```python
from build123d import *

# Parameters (mm, degrees)
MOUNTING_POINTS_DEPTH      = 116.951759253
MOUNTING_POINTS_DEPTH_BACK = 116.951759253
SKETCH3_R                  = 4.25
SKETCH3_R_2                = 12
SLOT_CLEARANCE_DEPTH       = 116.951759253
SLOT_CLEARANCE_DEPTH_BACK  = 116.951759253


with BuildPart() as part:
    # Sweep1: sweep along a path in Sketch1
    with BuildLine(Plane(origin=(0, 0, 0), x_dir=(1, 0, 0), z_dir=(0, 1, 0))) as sweep1_path:
        ThreePointArc((-100, -5), (0, 0), (100, -5))
    # Sketch2 → Sweep1 (sweep)
    with BuildSketch(Plane(origin=(0, 0, 0), x_dir=(0, 0, -1), z_dir=(1, 0, 0))):
        with BuildLine():
            Line((-37, 0), (37, 0))
            ThreePointArc((37, 0), (39.121320344, 0.878679656), (40, 3))
            Line((40, 3), (40, 15))
            Line((40, 15), (42, 15))
            Line((42, 15), (42, -2))
            Line((42, -2), (-42, -2))
            Line((-42, -2), (-42, 20))
            Line((-42, 20), (-40, 20))
            Line((-40, 20), (-40, 3))
            ThreePointArc((-40, 3), (-39.121320344, 0.878679656), (-37, 0))
        make_face()
    sweep(path=sweep1_path.line)

    # Sketch3 → Mounting points (cut, two sides: drawn at the far end of the back side and taken through both)
    with BuildSketch(Plane(origin=(0, 0, 0), x_dir=(1, 0, 0), z_dir=(0, 1, 0)).offset(-MOUNTING_POINTS_DEPTH_BACK)):
        with Locations(Location((0, 18, 0), (0, 0, 270))):
            Circle(SKETCH3_R)
        with Locations(Location((-77, -2.961481483, 0), (0, 0, 270))):
            Circle(SKETCH3_R_2)
        with Locations(Location((77, -2.961481483, 0), (0, 0, 270))):
            Circle(SKETCH3_R_2)
    extrude(amount=MOUNTING_POINTS_DEPTH + MOUNTING_POINTS_DEPTH_BACK, mode=Mode.SUBTRACT)

    # Sketch4 → Slot clearance (cut, two sides: drawn at the far end of the back side and taken through both)
    with BuildSketch(Plane(origin=(0, 0, 0), x_dir=(1, 0, 0), z_dir=(0, 1, 0)).offset(-SLOT_CLEARANCE_DEPTH_BACK)):
        with BuildLine():
            Line((-45, -17), (45, -17))
            ThreePointArc((45, -17), (50, -22), (45, -27))
            Line((45, -27), (-45, -27))
            ThreePointArc((-45, -27), (-50, -22), (-45, -17))
        make_face()
    extrude(amount=SLOT_CLEARANCE_DEPTH + SLOT_CLEARANCE_DEPTH_BACK, mode=Mode.SUBTRACT)


solid = part.part
```
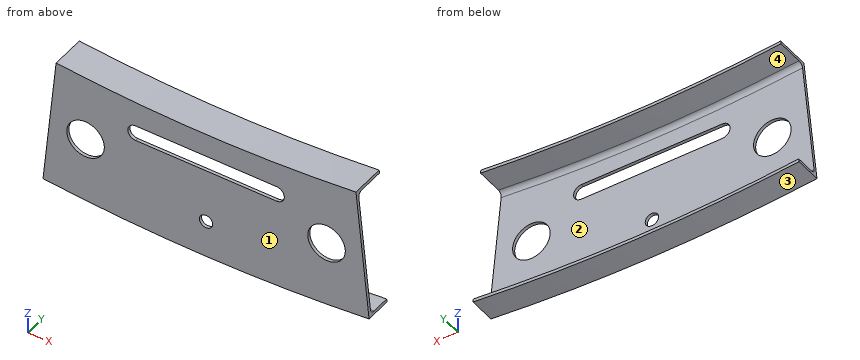
Input: part model. Units: mm. Frame: model coordinates. Face numbers are marked on the shaded views. Round coordinates to 2 decimals unless told otherwise and drop trailing zeros. Loops run counter-clockwise (first coordinate to the right, second up) from the corner with the lowest first, then second, coordinate; pieces in that order, holes last. Notation, with made-up numbers: M 62.25,-37 L 90.25,-37 A12 ccw 90.25,-20 Z; hole C 81,37.25 d3. An arc over 180 degrees is marked long. Answer in a Markdown table with one row per item. Add a question column.
1. Section B-B (x = 0). Output: boundary loops of the cut face in (y, z), and give its area (3 significant figures).
2. Section C-C (z = 19). Output: boundary loops of the cut face in (x, y).
3. Mould query, pull axis Z, two halves, no side actions, for the marked faces 1, 2, 3 and 4. Classes: released by +Z, released by -Z, zero draft, split by the parting line, or undercut.
4. Section A-A (y = 9.75). Output: boundary loops of the cut face in (x, z), and give its area (3 significant figures).
5. Contact query for flat-ended pins moving along their axis: pin 1 (10 mm diameter, centred on x = 0, z = -18, fed in from +Y); pin 2 (12 mm diameter, centred on y = 16, z = -29.5, fed in from +X); pin 3 (10 mm diameter, centred on y = 10.5, z = -26.5, fed in from -X); pin 4 (6 mm diameter, centred on x = 25, y = 5, fed in from +Z). Output: stop coordinate, or through.
6. Ray query, probe 1 along Y at (x, z) = (-11.5, -10.5); probe 2 along Z at (x, y) = (-50.5, 12.25); probe 3 along Z at (x, y) = (66.5, 14.5). Return the intervals inside material, ascending.
7. Section D-D (z = 5). Output: boundary loops of the cut face in (x, y), and give its area (3 significant figures).
Values follow:
| question | item | result |
|---|---|---|
| 1 | outline | M -2,-42 L 15,-42 L 15,-40 L 3,-40 A3 cw 0,-37 L 0,-22.25 L -2,-22.25 Z; M -2,-13.75 L 0,-13.75 L 0,17 L -2,17 Z; M -2,27 L 0,27 L 0,37 A3 cw 3,40 L 20,40 L 20,42 L -2,42 Z |
| 1 | area | 205 mm^2 |
| 2 | outline | M -98.6,-2 L -49,-2 L -49,0 L -98.6,0 Z; M 49,-2 L 98.6,-2 L 98.6,0 L 49,0 Z |
| 3 | face 1 | zero draft |
| 3 | face 2 | undercut |
| 3 | face 3 | released by -Z |
| 3 | face 4 | undercut |
| 4 | outline | M -104.19,-36.79 A1044.5 ccw 104.19,-36.79 L 103.99,-34.8 A1042.5 cw -103.99,-34.8 Z; M -96.01,44.8 A962.5 ccw 96.01,44.8 L 95.81,46.79 A960.5 cw -95.81,46.79 Z |
| 4 | area | 801 mm^2 |
| 5 | pin 1 | y = 0 |
| 5 | pin 2 | x = 104.05 |
| 5 | pin 3 | through |
| 5 | pin 4 | z = 42.41 |
| 6 | probe 1 | -2 to 0 |
| 6 | probe 2 | -40.78 to -38.78, 41.33 to 43.33 |
| 6 | probe 3 | -39.88 to -37.88, 42.3 to 44.3 |
| 7 | outline | M -100,-2 L -88.83,-2 L -88.83,0 L -100,0 Z; M -65.17,-2 L 65.17,-2 L 65.17,0 L -65.17,0 Z; M 88.83,-2 L 100,-2 L 100,0 L 88.83,0 Z |
| 7 | area | 305 mm^2 |
